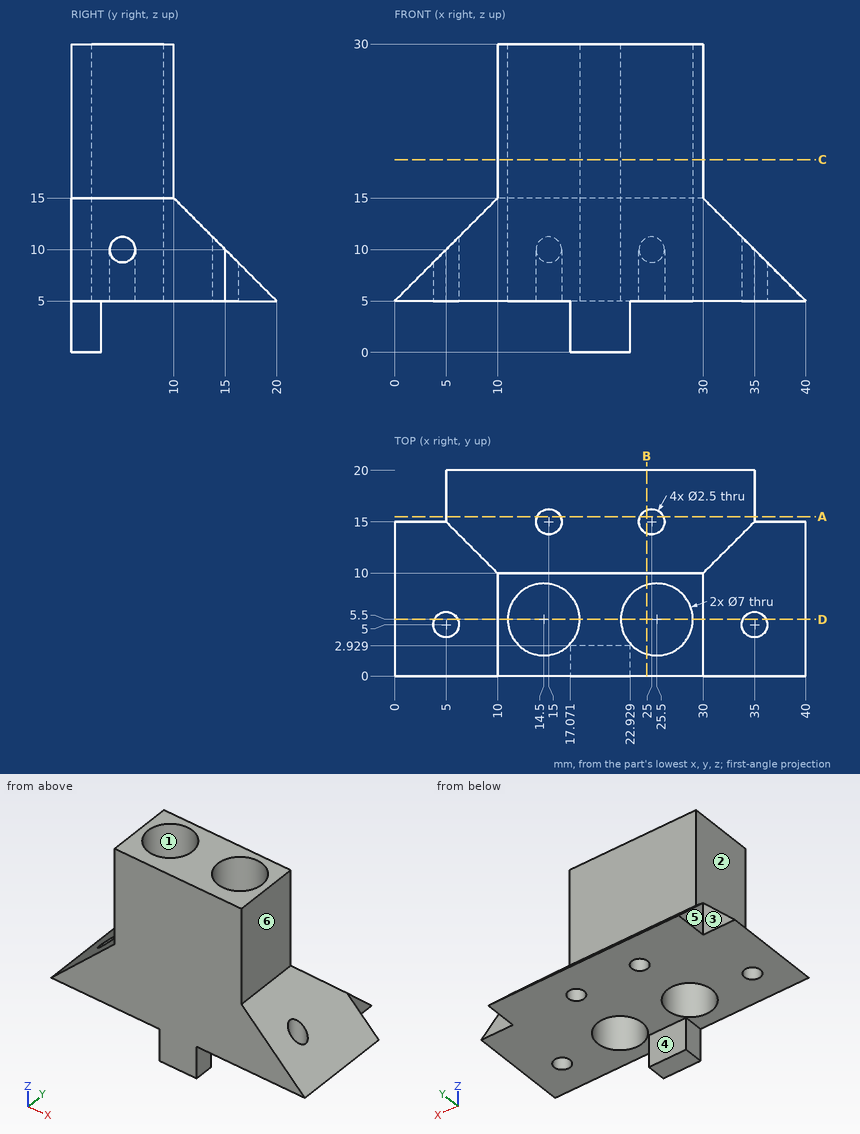
Design review of the part shown in the three views and the two pictorial views. Dimensions are in mm from the part's minimum x, y and z. A direction names the side the tool comes from. Coordinates: 2 decimals unless noted, no trailing zeros. Write each loop counter-clockwise with the first axis right and the second up, starting at its lowest first coordinate (ties: lowest second). Pieces come first, ordered by that corner, then holes. Notation, with made-up numbers: (-35, 47.25) -> (-19, 47.25) arc R19 cw to (-19, 58.25) -> close; hole circle Ø5 at (-17, -8.5). An arc over 180 degrees is marked (long way). Answer in a Markdown table with one row per item.
1. We need section D-D, the plane y = 5.5. State the section outline as (x, z) points, and give its area (3 significant figures).
Answers below:
| item | result |
|---|---|
| outline | (0, 5) -> (3.85, 5) -> (3.85, 8.85) -> close; (6.15, 5) -> (11, 5) -> (11, 30) -> (10, 30) -> (10, 15) -> (6.15, 11.15) -> close; (18, 5) -> (22, 5) -> (22, 30) -> (18, 30) -> close; (29, 5) -> (33.85, 5) -> (33.85, 11.15) -> (30, 15) -> (30, 30) -> (29, 30) -> close; (36.15, 5) -> (40, 5) -> (36.15, 8.85) -> close |
| area | 227 mm^2 |
2. Clearance check with flat-ended pins moving along their axes: pin 1 Ø1.5 at (x, z) = (37.5, 7) entering from +Y; pin 2 Ø5 at (y, z) = (6, 3) entering from -X; pin 3 Ø6 at (y, z) = (6.5, 21) entering from -X. State where each tip first meets the part, or that it passes through.
Answers below:
| item | result |
|---|---|
| pin 1 | stops at y = 15 |
| pin 2 | stops at x = 0 |
| pin 3 | stops at x = 10 |
3. We need section A-A, the plane y = 15.5. State the section outline as (x, z) points, and give its area (3 significant figures).
Answers below:
| item | result |
|---|---|
| outline | (5, 5) -> (13.85, 5) -> (13.85, 9.5) -> (5, 9.5) -> close; (16.15, 5) -> (23.85, 5) -> (23.85, 9.5) -> (16.15, 9.5) -> close; (26.15, 5) -> (35, 5) -> (35, 9.5) -> (26.15, 9.5) -> close |
| area | 114 mm^2 |
4. We need section B-B, the plane x = 24.5. State the section outline as (y, z) points.
Answers below:
| item | result |
|---|---|
| outline | (0, 5) -> (2.15, 5) -> (2.15, 30) -> (0, 30) -> close; (8.85, 5) -> (13.85, 5) -> (13.85, 11.15) -> (10, 15) -> (10, 30) -> (8.85, 30) -> close; (16.15, 5) -> (20, 5) -> (16.15, 8.85) -> close |
5. For the marked faces 4, 5 and 6, list the 3-axis set-ups (+Z, -Z, +X, -X, +Y, -Y) from which the entire face can be reached by the end or side of a thin tool; tool diameter is ignored.
Answers below:
| item | result |
|---|---|
| face 4 | -Z, +X, -X, +Y |
| face 5 | +Z, -Z, -X, +Y |
| face 6 | +Z, +X, +Y, -Y |
6. Wall thickness on probe 1 along X at (y, z) = (8.5, 23.25); probe 2 along X at (y, z) = (1.75, 19.75); probe 3 along Z at (x, y) = (28.5, 3.25): over which ranges is each line inside the solid? List them lowest first. Write a range as [from, to].
Answers below:
| item | result |
|---|---|
| probe 1 | x = [10, 12.7], [16.3, 23.7], [27.3, 30] |
| probe 2 | x = [10, 30] |
| probe 3 | z = [5, 30] |
7. Draft analysis for pull direction X (two halves, no side actions). For the marked faces 1, 2 and 3, state which applies: +X half, -X half, draft (parallel to the pull), parting line (faces both ways), or undercut.
Answers below:
| item | result |
|---|---|
| face 1 | undercut |
| face 2 | -X half |
| face 3 | draft |
8. We need section C-C, the plane z = 18.75. State the section outline as (x, y) points.
Answers below:
| item | result |
|---|---|
| outline | (10, 0) -> (30, 0) -> (30, 10) -> (10, 10) -> close; hole circle Ø7 at (14.5, 5.5); hole circle Ø7 at (25.5, 5.5) |
